Here's how the part is built. I have some questions about the finished solid (model axes, mm). A direction names the side the tool comes from. Coordinates: 2 decimals unless noted, no trailing zeros. Loops run counter-clockwise (first coordinate to the right, second up) from the corner with the lowest first, then second, coordinate; pieces in that order, holes last. Notation, with made-up numbers: (44, 72) - (51, 72) arc R24 cw to (51, 85) - close; hole circle Ø11 at (52.5, -35). An arc over 180 degrees is marked (long way). Use a Markdown table: item, result.
```python
from build123d import *

# Parameters (mm, degrees)
SKETCH1_W           = 4.5
SKETCH1_H           = 2
BOSS_EXTRUDE1_DEPTH = 35
BOSS_EXTRUDE2_START = 35
SKETCH1_3_R         = 1.5
SKETCH1_3_W         = 71.5
SKETCH1_3_H         = 24.5
BOSS_EXTRUDE2_DEPTH = 2
SKETCH1_5_W         = 4.5
SKETCH1_5_H         = 2
SKETCH3_R           = 2
CUT_EXTRUDE1_DEPTH  = 2
MOVE_FACE1_BY       = 0.05
MOVE_FACE1_2_BY     = 0.05
CUT_EXTRUDE2_DEPTH  = 85.017855245


with BuildPart() as part:
    # Sketch1 → Boss-Extrude1 (new, symmetric)
    with BuildSketch(Plane(origin=(0, 0, 0), x_dir=(1, 0, 0), z_dir=(0, 1, 0))):
        Polygon((-53, 25.5), (53, 25.5), (53, -25.5), (14, -25.5), (0, -25.5), (0, -27.5), (55, -27.5), (55, 27.5), (-55, 27.5), (-55, -27.5), (-4.5, -27.5), (-4.5, -25.5), (-14, -25.5), (-53, -25.5), align=None)
        with Locations((-2.25, -26.5)):
            Rectangle(SKETCH1_W, SKETCH1_H)
    extrude(amount=BOSS_EXTRUDE1_DEPTH, both=True)

    # Sketch1<3> → Boss-Extrude2 (add)
    with BuildSketch(Plane(origin=(0, 0, 0), x_dir=(1, 0, 0), z_dir=(0, 1, 0)).offset(BOSS_EXTRUDE2_START)):
        Polygon((53, -25.5), (53, 25.5), (-53, 25.5), (-53, -25.5), (-14, -25.5), (-4.5, -25.5), (0, -25.5), (14, -25.5), align=None)
        with Locations(Location((-37.5, -15.5, 0), (0, 0, 270))):
            Circle(SKETCH1_3_R, mode=Mode.SUBTRACT)
        with Locations(Location((37.5, -15.5, 0), (0, 0, 270))):
            Circle(SKETCH1_3_R, mode=Mode.SUBTRACT)
        Rectangle(SKETCH1_3_W, SKETCH1_3_H, mode=Mode.SUBTRACT)
        with Locations(Location((-37.5, 15.5, 0), (0, 0, 270))):
            Circle(SKETCH1_3_R, mode=Mode.SUBTRACT)
        with Locations(Location((37.5, 15.5, 0), (0, 0, 270))):
            Circle(SKETCH1_3_R, mode=Mode.SUBTRACT)
    extrude(amount=-BOSS_EXTRUDE2_DEPTH)

    # Sketch1<5> → Cut-Revolve1 (revolve, cut)
    with BuildSketch(Plane(origin=(0, 0, 0), x_dir=(1, 0, 0), z_dir=(0, 1, 0)), mode=Mode.PRIVATE) as cut_revolve1_sk:
        with Locations((-2.25, -26.5)):
            Rectangle(SKETCH1_5_W, SKETCH1_5_H)
    revolve(cut_revolve1_sk.sketch.rotate(Axis((0, 0, 6), (0, 0, -1)), 180), axis=Axis((0, 0, 6), (0, 0, -1)), mode=Mode.SUBTRACT)

    # Sketch3 → Cut-Extrude1 (cut)
    with BuildSketch(Plane.XY.offset(27.5)):
        with Locations((-17.5, -8.5)):
            Circle(SKETCH3_R)
        with Locations((17.5, -8.5)):
            Circle(SKETCH3_R)
    extrude(amount=-CUT_EXTRUDE1_DEPTH, mode=Mode.SUBTRACT)

    # Move Face1: a curved face moved outward by 0.05
    add(Solid.thicken(part.faces().sort_by_distance((15.5, -8.5, 26.5))[0], MOVE_FACE1_BY))

    # Move Face1 2: a curved face moved outward by 0.05
    add(Solid.thicken(part.faces().sort_by_distance((-19.5, -8.5, 26.5))[0], MOVE_FACE1_2_BY))

    # Sketch5 → Cut-Extrude2 (cut, through all)
    with BuildSketch(Plane(origin=(0, 0, 25.5), x_dir=(-1, 0, 0), z_dir=(0, 0, -1))):
        with BuildLine():
            Line((3.472963553, 19.69615506), (2.604722665, 14.772116295))
            ThreePointArc((2.604722665, 14.772116295), (5.500862492, 16.800015234), (3.472963553, 19.69615506))
        make_face()
        with BuildLine():
            ThreePointArc((-2.604722665, 14.772116295), (0, 15), (2.604722665, 14.772116295))
            Line((2.604722665, 14.772116295), (3.472963553, 19.69615506))
            ThreePointArc((3.472963553, 19.69615506), (0, 20), (-3.472963553, 19.69615506))
            Line((-3.472963553, 19.69615506), (-2.604722665, 14.772116295))
        make_face()
        with BuildLine():
            ThreePointArc((-3.472963553, 19.69615506), (-5.500862492, 16.800015234), (-2.604722665, 14.772116295))
            Line((-2.604722665, 14.772116295), (-3.472963553, 19.69615506))
        make_face()
    extrude(amount=-CUT_EXTRUDE2_DEPTH, mode=Mode.SUBTRACT)


solid = part.part
```
Q1. Which directions (+Z, -Z, +X, -X, +Y, -Y) give clear straight access to the entire face, cutting with the end or side of a thin tool? Please do faces 4 (the face through (-1, -1, -25.5)), 5 (the face through (1, 0, -27.5)), 6 (the face through (-3.32, -3.04, 26.49)).
Check values:
| item | result |
|---|---|
| face 4 | -Y |
| face 5 | -Z, +X, -X, +Y, -Y |
| face 6 | +Z |
Q2. I want a section at A-A, the plane y = -8.5. Write out the boundary of the cut face in (x, z).
Check values:
| item | result |
|---|---|
| outline | (-55, -27.5) - (55, -27.5) - (55, 27.5) - (19.45, 27.5) - (19.45, 25.5) - (53, 25.5) - (53, -25.5) - (-53, -25.5) - (-53, 25.5) - (-19.45, 25.5) - (-19.45, 27.5) - (-55, 27.5) - close; (-15.55, 25.5) - (15.55, 25.5) - (15.55, 27.5) - (-15.55, 27.5) - close |
Q3. Please list where these lines run through material, in increasing order: L1, parallel to Z at x = -33, y = 0; L2, parallel to Z at x = 37, y = 34; L3, parallel to X at y = 34, z = 15. Write a range as from..to.
Check values:
| item | result |
|---|---|
| L1 | -27.5..-25.5, 25.5..27.5 |
| L2 | -27.5..-16.91, -14.09..14.09, 16.91..27.5 |
| L3 | -55..-38.91, -36.09..36.09, 38.91..55 |
Q4. Will this pin go through, and if not, where does the flat tip stop? P1, Ø1.5, axis at x = 28.5, z = -14, coming from the -Y side.
Check values:
| item | result |
|---|---|
| P1 | y = 33 |
Q5. I want a section at D-D, the plane y = 27. Write out the boundary of the cut face in (x, z).
Check values:
| item | result |
|---|---|
| outline | (-55, -27.5) - (55, -27.5) - (55, 27.5) - (-55, 27.5) - close; hole (-53, -25.5) - (53, -25.5) - (53, 25.5) - (-53, 25.5) - close |
Q6. I want a section at B-B, the plane z = 0. Write out the boundary of the cut face in (x, y).
Check values:
| item | result |
|---|---|
| outline | (-55, -35) - (-53, -35) - (-53, 33) - (-35.75, 33) - (-35.75, 35) - (-55, 35) - close; (35.75, 33) - (53, 33) - (53, -35) - (55, -35) - (55, 35) - (35.75, 35) - close |
Q7. I want a section at C-C, the plane x = 0. Write out the boundary of the cut face in (y, z), then the cut area to 3 significant figures.
Check values:
| item | result |
|---|---|
| outline | (-35, -27.5) - (35, -27.5) - (35, -12.25) - (33, -12.25) - (33, -25.5) - (-35, -25.5) - close; (-35, 25.5) - (-4.5, 25.5) - (-4.5, 27.5) - (-35, 27.5) - close; (4.5, 25.5) - (15, 25.5) - (15, 27.5) - (4.5, 27.5) - close; (20, 25.5) - (33, 25.5) - (33, 12.25) - (35, 12.25) - (35, 27.5) - (20, 27.5) - close |
| area | 305 mm^2 |
Q8. If we mould it in two halves opening along X, with no side actions, what happens to faces 1 (the face through (55, 0, 0)), 2 (the face through (-1, 35, -13)), 3 (the face through (-53, -1, 0))? For each: pulls with the +X half, pulls with the -X half, needs draft (parallel to the pull), parting line crosses it, or undercut.
Check values:
| item | result |
|---|---|
| face 1 | pulls with the +X half |
| face 2 | needs draft |
| face 3 | undercut |
